Check sheet for the drawn part. Datum: minimum x, y, z corner. Units: mm. A direction names the side the tool comes from. Give positions to 0.01 mm unless a question says otherwise; leave off trailing zeros. Loops run counter-clockwise (first coordinate to the right, second up) from the corner with the lowest first, then second, coordinate; pieces in that order, holes last.
1. Cross-section at D-D, the plane z = 68. Record the cut outline in (x, y), plus the area to 3 significant figures.
2. Go/stop test with flat-tipped pins: pin 1 Ø22.5 at (x, z) = (26.5, 31) entering from +Y; pin 2 Ø12 at (x, y) = (38.5, 8) entering from -Z; pin 3 Ø5 at (y, z) = (6, 86.5) entering from -X; pin 4 Ø6 at (x, y) = (4.5, 15) entering from +Z. Record where each tip stops, or that it passes through.
3. Release check for a two-part mould opening along X. For the marked faces 1, 2 and 3 record: +X half, -X half, draft (parallel to the pull), parting line (faces both ways), or undercut.
4. Cross-section at A-A, the plane y = 6.75. Record the cut outline in (x, z).
5. Cross-section at C-C, the plane x = 24.5. Record the cut outline in (y, z).
6. Material ranges on L1, parallel to X at y = 17.5, z = 49; L2, parallel to Y at x = 33, z = 33.5; L3, parallel to Z at x = 8.5, y = 3.25 (1 decimal), recorded low to high.
7. Cross-section at B-B, the plane z = 56. Record the cut outline in (x, y).
8. Tool access check on the marked faces 4 and 5. Record the directions out of +Z, -Z, +X, -X, +Y, -Y that give a thin tool (end or side, any length) a straight path to the whole face; none if there is none.
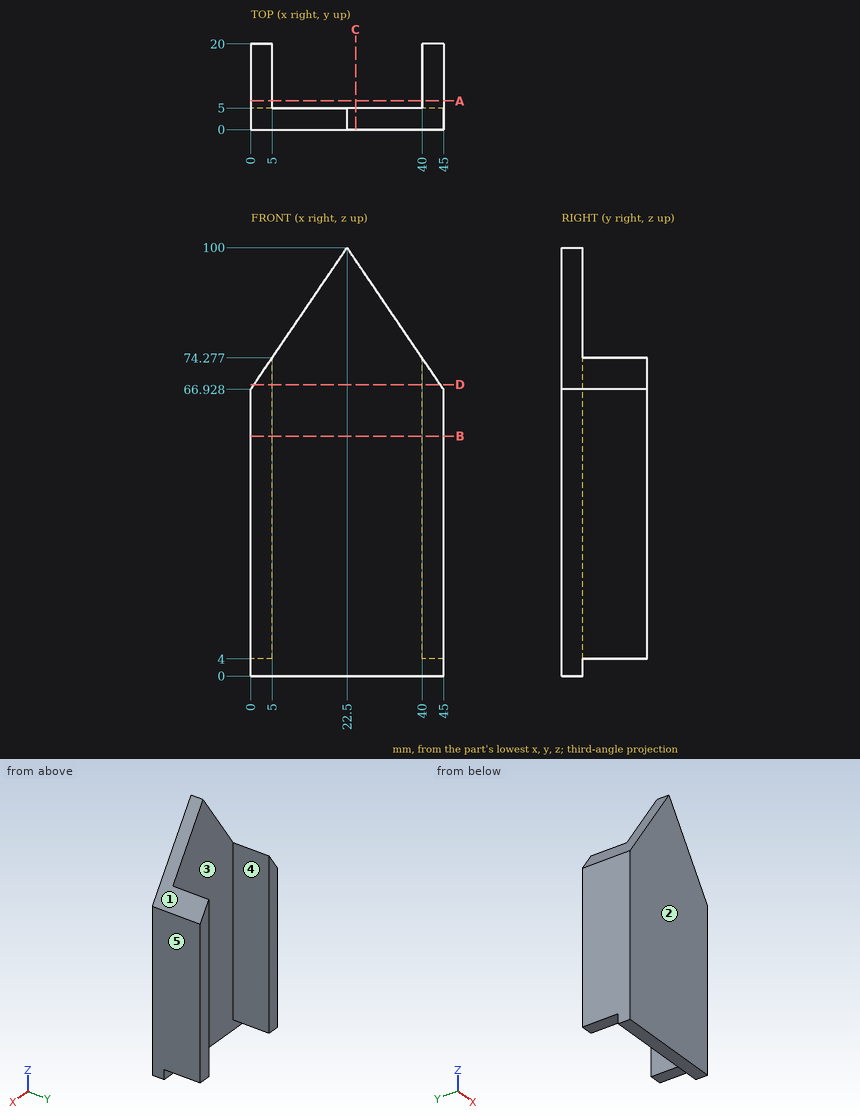
Result:
1. outline: (0.73, 0) - (44.27, 0) - (44.27, 20) - (40, 20) - (40, 5) - (5, 5) - (5, 20) - (0.73, 20) - close
1. area: 346 mm2
2. pin 1: stops at y = 5
2. pin 2: stops at z = 0
2. pin 3: stops at x = 11.76
2. pin 4: stops at z = 74.28
3. face 1: +X half
3. face 2: draft
3. face 3: undercut
4. outline: (0, 4) - (5, 4) - (5, 74.28) - (0, 66.93) - close; (40, 4) - (45, 4) - (45, 66.93) - (40, 74.28) - close
5. outline: (0, 0) - (5, 0) - (5, 97.06) - (0, 97.06) - close
6. L1: x = 0 to 5, 40 to 45
6. L2: y = 0 to 5
6. L3: z = 0 to 79.4
7. outline: (0, 0) - (45, 0) - (45, 20) - (40, 20) - (40, 5) - (5, 5) - (5, 20) - (0, 20) - close
8. face 4: +Z, -Z, +Y
8. face 5: +Z, -Z, +X, +Y, -Y
